Input: part model. Units: mm. Frame: model coordinates. A direction names the side the tool comes from. Coordinates: 2 decimals unless noted, no trailing zeros. Order: outer loops, then holes, each group sorted by start corner. A loop starts at its lowest first (then second) coordinate and runs counter-clockwise, first axis right, second up. Notation, with made-up numbers: M 58.25,-10 L 88.25,-10 A27 ccw 88.25,7 Z; hole C -18.75,36.5 d8. An arc over 180 degrees is marked long. Answer in a Markdown table with one row per item.
from build123d import *

# Parameters (mm, degrees)
SKETCH_1_W                 = 5.6
SKETCH_1_H                 = 4.2
EXTRUDE_1_DEPTH            = 1.4
SKETCH_3_W                 = 25.5
SKETCH_3_H                 = 0.3
SKETCH_3_W_2               = 5.6
EXTRUDE_2_DEPTH            = 0.2
PATTERN_START              = -2.1
PATTERN_LINEAR_1_OUTLINE_W = 5.6
PATTERN_LINEAR_1_OUTLINE_H = 1.4
PATTERN_LINEAR_1_DEPTH     = 4.2
SKETCH_4_W                 = 2.9
SKETCH_4_H                 = 1.1
SKETCH_4_H_2               = 0.55
CUT_EXTRUDE_1_DEPTH        = 0.2
SKETCH_5_W                 = 0.2
SKETCH_5_H                 = 0.8
EXTRUDE_3_DEPTH            = 0.8
SKETCH_6_W                 = 0.2
SKETCH_6_H                 = 0.8
EXTRUDE_4_DEPTH            = 0.8
SKETCH_7_W                 = 32.884134448
SKETCH_7_H                 = 1
EXTRUDE_5_DEPTH            = 0.2
CUT_EXTRUDE_START          = -1
SKETCH_8_W                 = 4.4
SKETCH_8_H                 = 3
CUT_EXTRUDE_2_DEPTH        = 1
SKETCH_9_W                 = 5.6
SKETCH_9_H                 = 4.2
EXTRUDE_6_DEPTH            = 0.6


# Read off the part's stored shape, not the designer's step: the pattern linear step
with BuildPart() as part:
    # Sketch 1 → Extrude 1 (new body)
    with BuildSketch(Plane.XY):
        Rectangle(SKETCH_1_W, SKETCH_1_H)
    extrude(amount=EXTRUDE_1_DEPTH)

    # Sketch 3 → Extrude 2 (add)
    with BuildSketch(Plane(origin=(0, 0, 0), x_dir=(-1, 0, 0), z_dir=(0, 0, -1))):
        Polygon((-2.8, 2.1), (2.8, 2.1), (2.8, 3.3), (-28.3, 3.3), (-28.3, 2.1), align=None)
        with Locations((-15.55, 1.95)):
            Rectangle(SKETCH_3_W, SKETCH_3_H)
        with Locations((0, 1.95)):
            Rectangle(SKETCH_3_W_2, SKETCH_3_H)
    extrude(amount=-EXTRUDE_2_DEPTH)

    # Pattern Linear 1 outline → Pattern Linear 1 (add)
    with BuildSketch(Plane(origin=(0, 0, 0), x_dir=(1, 0, 0), z_dir=(0, 1, 0)).offset(PATTERN_START)):
        with Locations((8.5, -0.7)):
            Rectangle(PATTERN_LINEAR_1_OUTLINE_W, PATTERN_LINEAR_1_OUTLINE_H)
        with Locations((17, -0.7)):
            Rectangle(PATTERN_LINEAR_1_OUTLINE_W, PATTERN_LINEAR_1_OUTLINE_H)
        with Locations((25.5, -0.7)):
            Rectangle(PATTERN_LINEAR_1_OUTLINE_W, PATTERN_LINEAR_1_OUTLINE_H)
    extrude(amount=PATTERN_LINEAR_1_DEPTH)

    # Sketch 4 → Cut-Extrude 1 (cut)
    with BuildSketch(Plane(origin=(0, 0, 0), x_dir=(-1, 0, 0), z_dir=(0, 0, -1))):
        with Locations((-4.25, 1.8)):
            Rectangle(SKETCH_4_W, SKETCH_4_H)
        with Locations((-12.75, 1.8)):
            Rectangle(SKETCH_4_W, SKETCH_4_H)
        with Locations((-21.25, 1.525)):
            Rectangle(SKETCH_4_W, SKETCH_4_H_2)
        with Locations((-21.25, 2.075)):
            Rectangle(SKETCH_4_W, SKETCH_4_H_2)
    extrude(amount=-CUT_EXTRUDE_1_DEPTH, mode=Mode.SUBTRACT)

    # Sketch 5 → Extrude 3 (add)
    with BuildSketch(Plane(origin=(28.3, 0, 0), x_dir=(0, 0, -1), z_dir=(1, 0, 0))):
        with Locations((-0.1, 2.9)):
            Rectangle(SKETCH_5_W, SKETCH_5_H)
    extrude(amount=EXTRUDE_3_DEPTH)

    # Sketch 6 → Extrude 4 (add)
    with BuildSketch(Plane.ZY.offset(2.8)):
        with Locations((0.1, 2.9)):
            Rectangle(SKETCH_6_W, SKETCH_6_H)
    extrude(amount=EXTRUDE_4_DEPTH)

    # Sketch 7 → Extrude 5 (add)
    with BuildSketch(Plane(origin=(0, 0, 0), x_dir=(-1, 0, 0), z_dir=(0, 0, -1))):
        with Locations((-12.798406479, -1.6)):
            Rectangle(SKETCH_7_W, SKETCH_7_H)
    extrude(amount=-EXTRUDE_5_DEPTH)

    # Sketch 8 → Cut-Extrude 2 (cut)
    with BuildSketch(Plane.XY.offset(1.4).offset(CUT_EXTRUDE_START)):
        Rectangle(SKETCH_8_W, SKETCH_8_H)
        with Locations((8.5, 0)):
            Rectangle(SKETCH_8_W, SKETCH_8_H)
        with Locations((17, 0)):
            Rectangle(SKETCH_8_W, SKETCH_8_H)
        with Locations((25.5, 0)):
            Rectangle(SKETCH_8_W, SKETCH_8_H)
    extrude(amount=-CUT_EXTRUDE_2_DEPTH, mode=Mode.SUBTRACT)

    # Sketch 9 → Extrude 6 (add)
    with BuildSketch(Plane.XY.offset(1.4)):
        Rectangle(SKETCH_9_W, SKETCH_9_H)
        with Locations((8.5, 0)):
            Rectangle(SKETCH_9_W, SKETCH_9_H)
        with Locations((17, 0)):
            Rectangle(SKETCH_9_W, SKETCH_9_H)
        with Locations((25.5, 0)):
            Rectangle(SKETCH_9_W, SKETCH_9_H)
    extrude(amount=EXTRUDE_6_DEPTH)


solid = part.part
1) Contact query for flat-ended pins moving along their axis: pin 1 (1.5 mm diameter, centred on x = -1, y = 0, fed in from -Z); pin 2 (2 mm diameter, centred on x = 18, y = -1, fed in from -Z); pin 3 (1 mm diameter, centred on x = 13, y = 1, fed in from -Z). Output: stop coordinate, or through.
Resolved:
| item | result |
|---|---|
| pin 1 | stops at z = 0.4 |
| pin 2 | stops at z = 0 |
| pin 3 | passes through |
2) Reachability of faces 3 (the face through (17, 0, 0.4)), 4 (the face through (4.3, -1.6, 0.2)), 5 (the face through (13, 3, 0.2)), 6 (the face through (28.8, -1.6, 0.2)) from +Z, -Z, +X, -X, +Y, -Y: full face, straight path, thin tool, end or side. Return the list, or none.
Resolved:
| item | result |
|---|---|
| face 3 | -Z |
| face 4 | +Z, +Y, -Y |
| face 5 | +Z, +X, -X, +Y |
| face 6 | +Z, +X, +Y, -Y |
3) Cut plane A-A, the plane z = 1.55. Output: boundary loops of the cut face in (x, y).
Resolved:
| item | result |
|---|---|
| outline | M -2.8,-2.1 L 2.8,-2.1 L 2.8,2.1 L -2.8,2.1 Z; M 5.7,-2.1 L 11.3,-2.1 L 11.3,2.1 L 5.7,2.1 Z; M 14.2,-2.1 L 19.8,-2.1 L 19.8,2.1 L 14.2,2.1 Z; M 22.7,-2.1 L 28.3,-2.1 L 28.3,2.1 L 22.7,2.1 Z |
4) Cut plane C-C, the plane x = 4. Output: boundary loops of the cut face in (y, z), and give its area (3 significant figures).
Resolved:
| item | result |
|---|---|
| outline | M -2.1,0 L -1.1,0 L -1.1,0.2 L -2.1,0.2 Z; M 2.35,0 L 3.3,0 L 3.3,0.2 L 2.35,0.2 Z |
| area | 0.390 mm2 |
5) Material intervals for probe 1 along X at (y, z) = (1.4, 0.45); probe 2 along Y at (x, z) = (21.5, 0.15); probe 3 along Y at (x, z) = (17, 1.6), sorted ascending.
Resolved:
| item | result |
|---|---|
| probe 1 | x = -2.8 to 2.8, 5.7 to 11.3, 14.2 to 19.8, 22.7 to 28.3 |
| probe 2 | y = -2.1 to -1.1, 2.35 to 3.3 |
| probe 3 | y = -2.1 to 2.1 |
6) Cut plane B-B, the plane y = 1. State how many separate pieces and enclosed holes the cut face has, and give its area (3 significant figures).
Resolved:
| item | result |
|---|---|
| separate pieces | 4 |
| enclosed holes | 0 |
| area | 37.8 mm2 |
7) Cut plane D-D, the plane x = 8.5. Output: boundary loops of the cut face in (y, z).
Resolved:
| item | result |
|---|---|
| outline | M -2.1,0 L -1.5,0 L -1.5,0.4 L 1.5,0.4 L 1.5,0 L 3.3,0 L 3.3,0.2 L 2.1,0.2 L 2.1,2 L -2.1,2 Z |
8) Mould query, pull axis X, two halves, no side actions, for faces 1 (the face through (0, 2.1, 1)), 2 (the face through (2.8, 0, 1)). Classes: +X half, -X half, draft (parallel to the pull), parting line (faces both ways), or undercut.
Resolved:
| item | result |
|---|---|
| face 1 | draft |
| face 2 | undercut |
